Input: part model. Units: mm. Frame: model coordinates. A direction names the side the tool comes from. Give positions to 0.01 mm unless a question says otherwise; leave off trailing zeros. Loops run counter-clockwise (first coordinate to the right, second up) from the corner with the lowest first, then second, coordinate; pieces in that order, holes last.
from build123d import *

# Parameters (mm, degrees)
CUT_EXTRUDE_1_DEPTH = 3
CUT_EXTRUDE_2_DEPTH = 3
CUT_REVOLVE_1_ANGLE = 15
CUT_REVOLVE_2_ANGLE = 15
CHAMFER_1_SIZE      = 1
CHAMFER_2_SIZE      = 1
FILLET_1_R          = 2
FILLET_2_R          = 2


with BuildPart() as part:
    # Эскиз2 → Повернуть1 (revolve)
    with BuildSketch(Plane(origin=(0, 0, 0), x_dir=(0, 0, -1), z_dir=(1, 0, 0))):
        Polygon((0, 30.25), (12, 30.25), (12, 26.25), (15, 26.25), (15, 34), (0, 34), align=None)
    revolve(axis=Axis((0, 0, 0), (0, 0, -1)))

    # Эскиз4 → Вырез-Вытянуть1 (cut)
    with BuildSketch(Plane(origin=(0, 34, 0), x_dir=(1, 0, 0), z_dir=(0, 1, 0))):
        with BuildLine():
            Line((3, 15), (3, 8))
            ThreePointArc((3, 8), (0, 5), (-3, 8))
            Line((-3, 8), (-3, 15))
            ThreePointArc((-3, 15), (0, 18), (3, 15))
        make_face()
    extrude(amount=-CUT_EXTRUDE_1_DEPTH, mode=Mode.SUBTRACT)

    # Эскиз5 → Вырез-Вытянуть2 (cut)
    with BuildSketch(Plane(origin=(0, -34, 0), x_dir=(-1, 0, 0), z_dir=(0, -1, 0))):
        with BuildLine():
            Line((3, 15), (3, 8))
            ThreePointArc((3, 8), (0, 5), (-3, 8))
            Line((-3, 8), (-3, 15))
            ThreePointArc((-3, 15), (0, 18), (3, 15))
        make_face()
    extrude(amount=-CUT_EXTRUDE_2_DEPTH, mode=Mode.SUBTRACT)

    # Эскиз8 → Вырез-Повернуть1 (revolve, cut)
    with BuildSketch(Plane(origin=(0, 0, 0), x_dir=(0, 0, -1), z_dir=(1, 0, 0))):
        Polygon((5, 34), (5, 31), (11, 31), (11, 34), (11, 37), (5, 37), align=None)
    revolve(axis=Axis((0, 0, 0), (0, 0, 1)), revolution_arc=CUT_REVOLVE_1_ANGLE, mode=Mode.SUBTRACT)

    # Эскиз9 → Вырез-Повернуть2 (revolve, cut)
    with BuildSketch(Plane(origin=(0, 0, 0), x_dir=(0, 0, -1), z_dir=(1, 0, 0))):
        Polygon((5, -34), (5, -31), (11, -31), (11, -34), (11, -37.830503046), (5, -37.830503046), align=None)
    revolve(axis=Axis((0, 0, 0), (0, 0, 1)), revolution_arc=CUT_REVOLVE_2_ANGLE, mode=Mode.SUBTRACT)

    # Фаска1
    chamfer_1_edges = [part.edges().sort_by_distance(p)[0] for p in [
        (3, 32.433694222, -15),
        (-3, 32.433694222, -15),
        (-3, -32.433694222, -15),
        (3, -32.433694222, -15),
    ]]
    chamfer(chamfer_1_edges, length=CHAMFER_1_SIZE)

    # Фаска2
    chamfer_2_edges = [part.edges().sort_by_distance(p)[0] for p in [
        (-3, 32.433694222, -11),
        (3, -32.433694222, -11),
    ]]
    chamfer(chamfer_2_edges, length=CHAMFER_2_SIZE)

    # Скругление1
    fillet_1_edges = [part.edges().sort_by_distance(p)[0] for p in [
        (8.411618966, -31.392589354, -5),
        (8.411618966, -31.392589354, -11),
    ]]
    fillet(fillet_1_edges, radius=FILLET_1_R)

    # Скругление2
    fillet_2_edges = [part.edges().sort_by_distance(p)[0] for p in [
        (-8.411618966, 31.392589354, -5),
        (-8.411618966, 31.392589354, -11),
    ]]
    fillet(fillet_2_edges, radius=FILLET_2_R)


solid = part.part
(1) Mould query, pull axis X, two halves, no side actions, for faces 5 (the flat face through (-20, -23, 0)), 6 (the flat face through (5, -32, -11)), 7 (the flat face through (-5, 32, -11)), 8 (the cylindrical face through (10.21, 32.43, -7.4)). Classes: +X half, -X half, draft (parallel to the pull), parting line (faces both ways), or undercut.
Values follow:
face 5: draft
face 6: undercut
face 7: undercut
face 8: parting line
(2) Cut plane A-A (y = 0). Return the cut outline in (x, z).
Values follow:
outline: (-34, -15) - (-26.25, -15) - (-26.25, -12) - (-30.25, -12) - (-30.25, 0) - (-34, 0) - close; (26.25, -15) - (34, -15) - (34, 0) - (30.25, 0) - (30.25, -12) - (26.25, -12) - close
(3) Cut plane B-B (x = 10.5). Return the cut outline in (y, z).
Values follow:
outline: (-32.34, -15) - (-24.06, -15) - (-24.06, -12) - (-28.37, -12) - (-28.37, 0) - (-32.34, 0) - close; (24.06, -15) - (32.34, -15) - (32.34, 0) - (28.37, 0) - (28.37, -12) - (24.06, -12) - close
(4) Reachability of faces 1 (the flat face through (-3, -32, -11)), 2 (the cylindrical face through (7.83, -31.54, -5.57)), 3 (the flat face through (-3, 32, -13)), 4 (the flat face through (25, -9, -12)) from +Z, -Z, +X, -X, +Y, -Y: full face, straight path, thin tool, end or side. Return the list, or none.
Values follow:
face 1: -Z, -Y
face 2: -Y
face 3: -Z, +Y
face 4: +Z
(5) Cut plane D-D (x = 27.5). Return the cut outline in (y, z), and give its area (3 significant figures).
Values follow:
outline: (-19.99, -15) - (19.99, -15) - (19.99, 0) - (12.6, 0) - (12.6, -12) - (-12.6, -12) - (-12.6, 0) - (-19.99, 0) - close
area: 297 mm2
(6) Cut plane C-C (z = -1.75). Return the cut outline in (x, y).
Values follow:
outline: circle Ø68 at (0, 0); hole circle Ø60.5 at (0, 0)
(7) Pin query (flat end, axial travel): pin 1 Ø6.5 at (x, z) = (0, -8.5) entering from +Y; pin 2 Ø2.5 at (y, z) = (-32.5, -11.5) entering from +X; pin 3 Ø1.5 at (x, z) = (-4, -8) entering from -Y. Return the tip coordinate at first contact, or that it passes through.
Values follow:
pin 1: stops at y = 33.89
pin 2: stops at x = 13.4
pin 3: stops at y = -33.84
(8) Ray query, probe 1 along X at (y, z) = (0, -13.9); probe 2 along X at (y, z) = (0, -6); probe 3 along Y at (x, z) = (12, -8.75). Return the intervals inside material, ascending.
Values follow:
probe 1: x = -34 to -26.25, 26.25 to 34
probe 2: x = -34 to -30.25, 30.25 to 34
probe 3: y = -31.81 to -27.77, 27.77 to 31.81
